The figure shows three views and two pictorial views of one solid part (mm, origin at its lowest corner). Answer the questions. A direction names the side the tool comes from. Give positions to 0.01 mm unless a question says otherwise; leave off trailing zeros. Order: outer loops, then holes, each group sorted by start corner. A loop starts at its lowest first (then second) coordinate and runs counter-clockwise, first axis right, second up. Notation, with made-up numbers: (42, 29.5) - (88, 29.5) arc R12 cw to (88, 48.5) - close; hole circle Ø3 at (5.5, -33.5). An arc over 180 degrees is marked (long way). Use a Markdown table: item, result. Add a question column.
1. Consider L1, parallel to Z at x = 43.36, y = 0.5 (3 decimals); L2, parallel to X at y = 0.5, z = 16.52 (3 decimals); L3, parallel to Y at x = 35.5, z = 8.5. Determine where each line is inside the solid, lowest interval first.
2. Flat-ended cylindrical pins translate along their axes: P1, Ø1.2, axis at y = 4, z = 8.5, coming from the +X side; P2, Ø9, axis at x = 16, z = 10.5, coming from the +Y side; P3, Ø1.5, axis at x = 43.36, z = 1.28, coming from the -Y side; P4, Ø1.3, axis at y = 0.5, z = 6, coming from the -X side. Find the tip coordinate at first contact, or state that the pin passes through.
3. A cutting plane is placed at C-C on x = 5.5. Determine the outline of the cut face in (y, z), and give its area (3 significant figures).
4. A cutting plane is placed at B-B on z = 16.52. Determine the outline of the cut face in (x, y) (3 decimals).
5. A cutting plane is placed at A-A on x = 43.36. Determine the outline of the cut face in (y, z) (3 decimals), and give its area (3 significant figures).
6. Which of the six approach directions +Z, -Z, +X, -X, +Y, -Y give full straight-line access (tool end or side, diameter ignored) to the marked faces 1, 2 and 3?
7. A cutting plane is placed at D-D on z = 9.5. Determine the outline of the cut face in (x, y), and give its area (3 significant figures).
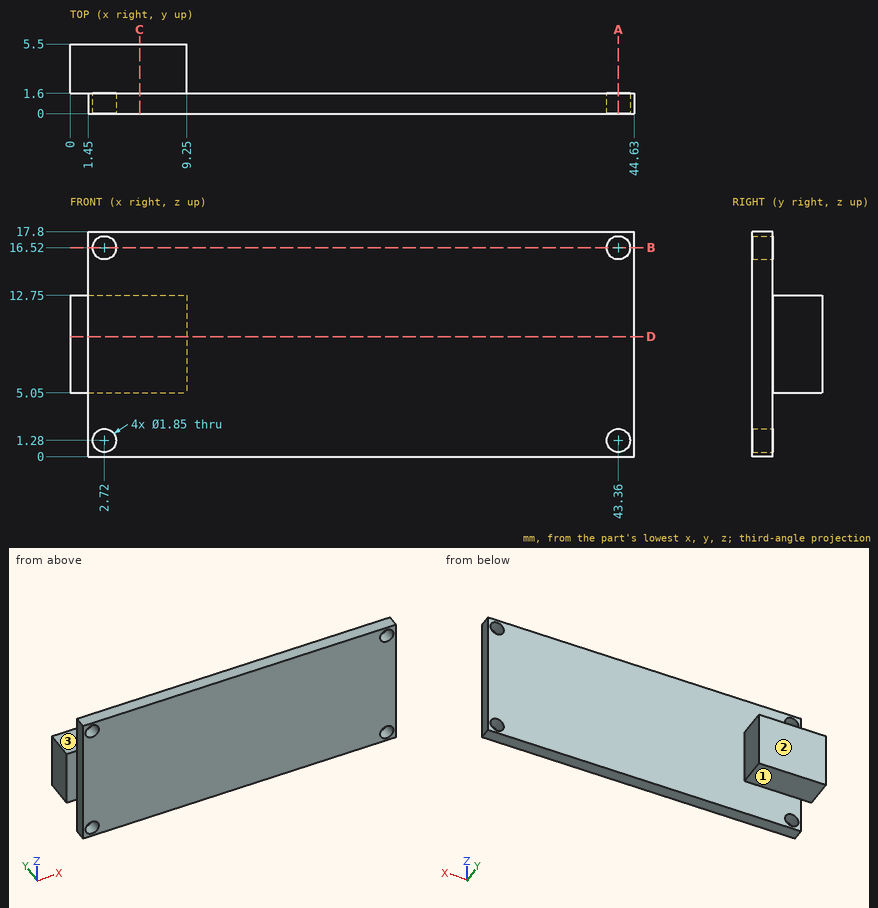
Output values:
| question | item | result |
|---|---|---|
| 1 | L1 | 0 to 0.355, 2.205 to 15.595, 17.445 to 17.8 |
| 1 | L2 | 1.45 to 1.795, 3.645 to 42.435, 44.285 to 44.63 |
| 1 | L3 | 0 to 1.6 |
| 2 | P1 | x = 9.25 |
| 2 | P2 | y = 1.6 |
| 2 | P3 | through |
| 2 | P4 | x = 1.45 |
| 3 | outline | (0, 0) - (1.6, 0) - (1.6, 5.05) - (5.5, 5.05) - (5.5, 12.75) - (1.6, 12.75) - (1.6, 17.8) - (0, 17.8) - close |
| 3 | area | 58.5 mm² |
| 4 | outline | (1.45, 0) - (1.795, 0) - (1.795, 1.6) - (1.45, 1.6) - close; (3.645, 0) - (42.435, 0) - (42.435, 1.6) - (3.645, 1.6) - close; (44.285, 0) - (44.63, 0) - (44.63, 1.6) - (44.285, 1.6) - close |
| 5 | outline | (0, 0) - (1.6, 0) - (1.6, 0.355) - (0, 0.355) - close; (0, 2.205) - (1.6, 2.205) - (1.6, 15.595) - (0, 15.595) - close; (0, 17.445) - (1.6, 17.445) - (1.6, 17.8) - (0, 17.8) - close |
| 5 | area | 22.6 mm² |
| 6 | face 1 | -Z, +X, -X, +Y |
| 6 | face 2 | +Z, -Z, +X, -X, +Y |
| 6 | face 3 | +Z, +X, -X, +Y |
| 7 | outline | (0, 1.6) - (1.45, 1.6) - (1.45, 0) - (44.63, 0) - (44.63, 1.6) - (9.25, 1.6) - (9.25, 5.5) - (0, 5.5) - close |
| 7 | area | 105 mm² |
